Autodesk Inventor part; units mm, degrees
ref_plane "YZ Plane" through (0, 0, 0) normal (1, 0, 0) x (0, 1, 0)
ref_plane "XZ Plane" through (0, 0, 0) normal (0, 1, 0) x (-1, 0, 0)
ref_plane "XY Plane" through (0, 0, 0) normal (0, 0, 1) x (1, 0, 0)
sketch "Sketch1" plane through (0, 0, 0) normal (0, 1, 0) x (-1, 0, 0)
  line L0 (0, -7.3323) -> (-6.35, -3.6662)
  line L1 (-6.35, -3.6662) -> (-6.35, 3.6662)
  line L2 (-6.35, 3.6662) -> (0, 7.3323)
  line L3 (0, 7.3323) -> (6.35, 3.6662)
  line L4 (6.35, 3.6662) -> (6.35, -3.6662)
  line L5 (6.35, -3.6662) -> (0, -7.3323)
  point P0 (0, 0)
  dimension "d19" = 12.7
extrude "Extrusion1" add sketch "Sketch1" along normal blind 170
sketch "Sketch5" plane through (0, 170, 0) normal (0, 1, 0) x (1, 0, 0)
  point P0 (0, 0)
  point P1 (0, 0)
hole "Hole3" at (0, 170, 0) direction (0, -1, 0) diameter 4.134 depth 14.2 tip angle 118
sketch "Sketch6" plane through (0, 0, 0) normal (0, -1, 0) x (1, 0, 0)
  point P0 (0, 0)
  point P1 (0, 0)
hole "Hole4" at (0, 0, 0) direction (0, 1, 0) diameter 4.134 depth 14.2 tip angle 118
properties part number "Adapter Standoff"
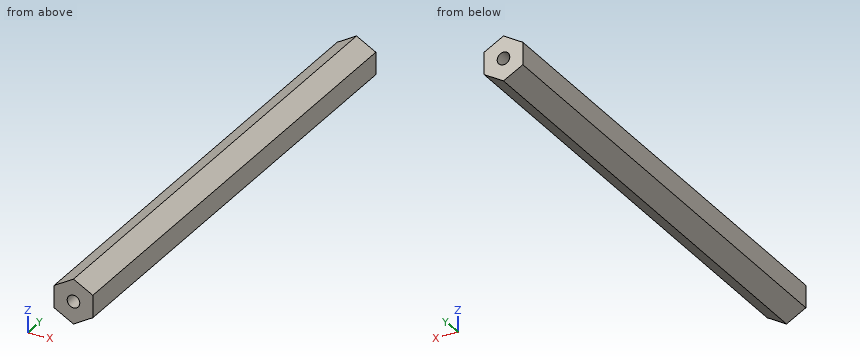
Here's how the part is built. I have some questions about the finished solid (model axes, mm). Give positions to 0.01 mm unless a question says otherwise; leave off trailing zeros. Loops run counter-clockwise (first coordinate to the right, second up) from the corner with the lowest first, then second, coordinate; pieces in that order, holes last. Notation, with made-up numbers: (65.5, 11) -> (78.5, 11) arc R13 ccw to (78.5, 33) -> close; hole circle Ø9 at (-24.5, -14.5). An arc over 180 degrees is marked (long way). One line per item, written item: value.
Q1. Suppose I cut it at A-A on y = 113.5. Please give me the cut outline in (x, z).
Answers follow:
outline: (-6.35, -3.67) -> (0, -7.33) -> (6.35, -3.67) -> (6.35, 3.67) -> (0, 7.33) -> (-6.35, 3.67) -> close
Q2. If I drill on line 1 along Z through (x, y) = (0, 3.5); line 2 along X through (y, z) = (7.5, 0); line 3 along Z through (x, y) = (0.75, 7.5), over which ranges is the centre line in solid material (lowest first)?
Answers follow:
line 1: -7.33 to -2.07, 2.07 to 7.33
line 2: -6.35 to -2.07, 2.07 to 6.35
line 3: -6.9 to -1.93, 1.93 to 6.9
Q3. I'm going to push a flat-ended pin straight in: pin 1 Ø5 at (x, y) = (0.5, 115.5) entering from +Z. Where does the tip first touch, or does it pass through?
Answers follow:
pin 1: z = 7.33
